from build123d import *

# Parameters (mm, degrees)
SKETCH1_R           = 29.5
SKETCH1_R_2         = 3
BOSS_EXTRUDE1_DEPTH = 4
SKETCH2_R           = 10
SKETCH2_R_2         = 5
BOSS_EXTRUDE2_DEPTH = 16
SKETCH3_R           = 3
CUT_EXTRUDE1_DEPTH  = 13


with BuildPart() as part:
    # Sketch1 → Boss-Extrude1 (new body)
    with BuildSketch(Plane(origin=(0, 0, 0), x_dir=(1, 0, 0), z_dir=(0, 1, 0))):
        with Locations(Location((0, 0, 0), (0, 0, 270))):
            Circle(SKETCH1_R)
        with Locations(Location((-16.263455967, 16.263455967, 0), (0, 0, 270))):
            Circle(SKETCH1_R_2, mode=Mode.SUBTRACT)
        with Locations(Location((5.932823239, 22.141597761, 0), (0, 0, 270))):
            Circle(SKETCH1_R_2, mode=Mode.SUBTRACT)
        with Locations(Location((22.121582963, 5.858126996, 0), (0, 0, 270))):
            Circle(SKETCH1_R_2, mode=Mode.SUBTRACT)
        with Locations(Location((16.11406348, -16.303485564, 0), (0, 0, 270))):
            Circle(SKETCH1_R_2, mode=Mode.SUBTRACT)
        with Locations(Location((-6.082215726, -22.181627357, 0), (0, 0, 270))):
            Circle(SKETCH1_R_2, mode=Mode.SUBTRACT)
        with Locations(Location((-22.27097545, -5.898156592, 0), (0, 0, 270))):
            Circle(SKETCH1_R_2, mode=Mode.SUBTRACT)
    extrude(amount=BOSS_EXTRUDE1_DEPTH)

    # Sketch2 → Boss-Extrude2 (add)
    with BuildSketch(Plane(origin=(0, 4, 0), x_dir=(1, 0, 0), z_dir=(0, 1, 0))):
        with Locations(Location((0, 0, 0), (0, 0, 270))):
            Circle(SKETCH2_R)
        with Locations(Location((0, 0, 0), (0, 0, 270))):
            Circle(SKETCH2_R_2, mode=Mode.SUBTRACT)
    extrude(amount=BOSS_EXTRUDE2_DEPTH)

    # Sketch3 → Cut-Extrude1 (cut, symmetric)
    with BuildSketch(Plane.XY):
        with Locations((0, 12)):
            Circle(SKETCH3_R)
    extrude(amount=CUT_EXTRUDE1_DEPTH, both=True, mode=Mode.SUBTRACT)


solid = part.part
Model file for the job. Use its own axes, mm. A direction names the side the tool comes from. Round coordinates to 2 decimals unless told otherwise and drop trailing zeros. Loops run counter-clockwise (first coordinate to the right, second up) from the corner with the lowest first, then second, coordinate; pieces in that order, holes last. Notation, with made-up numbers: M 72,-29.5 L 121,-29.5 A15 ccw 121,-18.5 Z; hole C -22.5,73 d6. An arc over 180 degrees is marked long. One line per question, with ' | ' between items.
1) Mould opens along Z. For faces 3 (the cylindrical face through (-3.83, 11.888, 9.237)), 4 (the cylindrical face through (-3.55, 1.97, 23.79)), 5 (the flat face through (0, 0, 0)) say: +Z half, -Z half, draft (parallel to the pull), parting line (faces both ways), or undercut.
Solved:
face 3: parting line | face 4: undercut | face 5: draft
2) Flat gauge pins, fed straight in: pin 1 (10 mm diameter, centred on y = 10, z = 4, fed in from +X); pin 2 (9.5 mm diameter, centred on x = -16.26, z = -16.26, fed in from +Y); pin 3 (5.5 mm diameter, centred on x = 16.11, z = 16.3, fed in from +Y); pin 4 (4 mm diameter, centred on x = -15, y = 3.5, fed in from -Z). Where does each tip first touch, or does it go through?
Solved:
pin 1: stops at x = 10 | pin 2: stops at y = 4 | pin 3: passes through | pin 4: stops at z = -26.48
3) Band-saw the part on C-C (z = -23.5). Give the cut face in (x, y).
Solved:
outline: M -17.83,0 L 3.26,0 L 3.26,4 L -17.83,4 Z; M 8.61,0 L 17.83,0 L 17.83,4 L 8.61,4 Z
4) 3-axis set-ups, long thin cutter, end or side, ignore diameter. For faces 1 (the cylindrical face through (-0.65, 9.07, 7.04)), 2 (the flat face through (-13, 4, 0)): which of +Z, -Z, +X, -X, +Y, -Y reach the whole face in a straight line?
Solved:
face 1: +Z, -Z | face 2: +Y
5) Band-saw the part on A-A (x = 0). Give the cut face in (y, z), then the cut area to 3 significant figures.
Solved:
outline: M 0,-29.5 L 4,-29.5 L 4,-10 L 9,-10 L 9,-5 L 4,-5 L 4,5 L 9,5 L 9,10 L 4,10 L 4,29.5 L 0,29.5 Z; M 15,-10 L 20,-10 L 20,-5 L 15,-5 Z; M 15,5 L 20,5 L 20,10 L 15,10 Z | area: 336 mm²
6) Band-saw the part on B-B (y = 12). Give the cut face in (x, z), then the cut area to 3 significant figures.
Solved:
outline: M -3,-9.54 L -3,-4 A5 cw -3,4 L -3,9.54 A10 ccw Z; M 3,-9.54 A10 ccw 3,9.54 L 3,4 A5 cw 3,-4 Z | area: 174 mm²
7) Band-saw the part on D-D (y = 5.75). Give the cut face in (x, z), then the cut area to 3 significant figures.
Solved:
outline: C 0,0 d20; hole C 0,0 d10 | area: 236 mm²
8) Drill centre lines: line 1 along X through (y, z) = (16, 0); line 2 along Y through (x, z) = (-17, -2); line 3 along X through (y, z) = (2.5, 24.5). Where is each one in solid material? Low to high.
Solved:
line 1: x = -10 to -5, 5 to 10 | line 2: y = 0 to 4 | line 3: x = -16.43 to -7.99, -4.18 to 16.43
